Here's how the part is built. I have some questions about the finished solid (model axes, mm). Coordinates: 2 decimals unless noted, no trailing zeros. Write each loop counter-clockwise with the first axis right and the second up, starting at its lowest first coordinate (ties: lowest second). Pieces come first, ordered by that corner, then holes.
```python
from build123d import *

# Parameters (mm, degrees)
BOSS_EXTRUDE1_DEPTH = 4


with BuildPart() as part:
    # Sketch1 → Boss-Extrude1 (new body)
    with BuildSketch(Plane(origin=(0, 0, 0), x_dir=(1, 0, 0), z_dir=(0, 1, 0))):
        Polygon((-219.316556264, 100.420860934), (-223.316556264, 100.420860934), (-223.316556264, -99.579139066), (-219.316556264, -99.579139066), (-219.316556264, -220.579139066), (-98.316556264, -220.579139066), (-98.316556264, -224.579139066), (101.683443736, -224.579139066), (101.683443736, -220.579139066), (222.683443736, -220.579139066), (222.683443736, -99.579139066), (226.683443736, -99.579139066), (226.683443736, 100.420860934), (222.683443736, 100.420860934), (222.683443736, 221.420860934), (101.683443736, 221.420860934), (101.683443736, 225.420860934), (-98.316556264, 225.420860934), (-98.316556264, 221.420860934), (-219.316556264, 221.420860934), align=None)
        Polygon((-179.316556264, -180.579139066), (-98.316556264, -180.579139066), (-98.316556264, -184.579139066), (101.683443736, -184.579139066), (101.683443736, -180.579139066), (182.683443736, -180.579139066), (182.683443736, -99.579139066), (186.683443736, -99.579139066), (186.683443736, 100.420860934), (182.683443736, 100.420860934), (182.683443736, 181.420860934), (101.683443736, 181.420860934), (101.683443736, 185.420860934), (-98.316556264, 185.420860934), (-98.316556264, 181.420860934), (-179.316556264, 181.420860934), (-179.316556264, 100.420860934), (-183.316556264, 100.420860934), (-183.316556264, -99.579139066), (-179.316556264, -99.579139066), align=None, mode=Mode.SUBTRACT)
    extrude(amount=BOSS_EXTRUDE1_DEPTH)


solid = part.part
```
1) Imagine slicing it at C-C on z = -198. Please give me the cut outline in (x, y), then the cut area to 3 significant figures.
Values follow:
outline: (-219.32, 0) - (222.68, 0) - (222.68, 4) - (-219.32, 4) - close
area: 1,770 mm2
2) Imagine slicing it at A-A on z = 31.5. Please give me the cut outline in (x, y), then the cut area to 3 significant figures.
Values follow:
outline: (-223.32, 0) - (-183.32, 0) - (-183.32, 4) - (-223.32, 4) - close; (186.68, 0) - (226.68, 0) - (226.68, 4) - (186.68, 4) - close
area: 320 mm2
3) Imagine slicing it at D-D on x = -191. Please give me the cut outline in (y, z).
Values follow:
outline: (0, -221.42) - (4, -221.42) - (4, 220.58) - (0, 220.58) - close
4) Imagine slicing it at B-B on x = 125.5. Please give me the cut outline in (y, z).
Values follow:
outline: (0, -221.42) - (4, -221.42) - (4, -181.42) - (0, -181.42) - close; (0, 180.58) - (4, 180.58) - (4, 220.58) - (0, 220.58) - close
5) Will these pins go through, and if not, where does the flat tip stop? pin 1 (2 mm diameter, centred on x = 184.5, y = 2, fed in from +Z); pin 2 (1 mm diameter, centred on y = 3.5, z = -135.5, fed in from -X); pin 3 (1.2 mm diameter, centred on y = 3, z = 153.5, fed in from +X).
Values follow:
pin 1: stops at z = 220.58
pin 2: stops at x = -219.32
pin 3: stops at x = 222.68
6) I need wall thicknesses on probe 1 along Z at (x, y) = (-131, 3.15); probe 2 along X at (y, z) = (2.1, 132); probe 3 along X at (y, z) = (3.85, -7). Which ranges of each line are inside material? Lowest first, please.
Values follow:
probe 1: z = -221.42 to -181.42, 180.58 to 220.58
probe 2: x = -219.32 to -179.32, 182.68 to 222.68
probe 3: x = -223.32 to -183.32, 186.68 to 226.68
